The listing builds one solid part. Answer for the finished solid, in the listing's coordinates (mm). A direction names the side the tool comes from. Give positions to 0.01 mm unless a question says otherwise; leave off trailing zeros. Order: outer loops, then holes, each group sorted by start corner. A loop starts at its lowest first (then second) coordinate and runs counter-clockwise, first axis right, second up. Notation, with made-up numbers: (46.25, -27.5) - (50.25, -27.5) arc R22 ccw to (50.25, 8.5) - close; hole circle Ø9 at (13, 47.25). An arc over 180 degrees is marked (long way). Answer as a JSON object with one key per item and string values. Group by question number.
Q1. A cutting plane is placed at B-B, the plane y = 10. Give the vertices of the cut face in (x, z).
Q2. A cutting plane is placed at D-D, the plane y = -5. Give the vertices of the cut face in (x, z).
Q3. The mould has two halves that part along Y. Classify faces 1 (the face through (0, 19, 9)), 2 (the face through (-19.02, -11.06, 3.08)), 3 (the face through (7.706, -4.7, -1.521)): released by +Y, released by -Y, zero draft, split by the parting line, or undercut.
Q4. Given pin 1 (10.5 mm diameter, centred on x = 0, y = 0, fed in from +Z); pin 2 (2 mm diameter, centred on x = 10.5, z = 6.5, fed in from -Y); pin 3 (3.5 mm diameter, centred on y = 17.5, z = 2, fed in from -X); pin 4 (4 mm diameter, centred on y = -8.5, z = 0, fed in from -X), each flat-ended and moving along its own axis, determine where each tip first touches the part or whether it passes through.
Q5. A cutting plane is placed at A-A, the plane z = 7.75. Give the vertices of the cut face in (x, y).
Q6. For faces 4 (the face through (-15, -8, 4)), 5 (the face through (0, 17, 4)), 6 (the face through (-12.906, -13.225, 1.583)), 7 (the face through (-5, 18, 2)), determine the directions among +Z, -Z, +X, -X, +Y, -Y from which every point of the face is accessible in a straight line to the end or side of a thin tool.
Q7. A cutting plane is placed at C-C, the plane x = 0. Give the vertices of the cut face in (y, z), and give its area (3 significant figures).
Q8. Consider line 1 (Y direction, x = 0, z = -0.75); line 2 (Z direction, x = 15.5, y = -5); line 3 (X direction, y = -10.5, z = 3). Determine where each line is inside the solid, lowest interval first.
from build123d import *

# Parameters (mm, degrees)
SKETCH_1_R          = 22
SKETCH_1_R_2        = 17
EXTRUDE_1_DEPTH     = 9
SKETCH_2_R          = 22
EXTRUDE_2_DEPTH     = 3
SKETCH_3_R          = 1
CUT_EXTRUDE_1_DEPTH = 3
CUT_EXTRUDE_2_DEPTH = 25
SKETCH_5_R          = 4
CUT_EXTRUDE_3_DEPTH = 10
FILLET_1_R          = 10
FILLET_2_R          = 10


with BuildPart() as part:
    # 草图1 → 凸台-拉伸1 (new body)
    with BuildSketch(Plane.XY):
        Circle(SKETCH_1_R)
        Circle(SKETCH_1_R_2, mode=Mode.SUBTRACT)
    extrude(amount=EXTRUDE_1_DEPTH)

    # 草图2 → 凸台-拉伸2 (add)
    with BuildSketch(Plane(origin=(0, 0, 0), x_dir=(-1, 0, 0), z_dir=(0, 0, -1))):
        Circle(SKETCH_2_R)
    extrude(amount=EXTRUDE_2_DEPTH)

    # 草图3 → 切除-拉伸1 (cut)
    with BuildSketch(Plane(origin=(0, 0, -3), x_dir=(-1, 0, 0), z_dir=(0, 0, -1))):
        with Locations((0, 10)):
            Circle(SKETCH_3_R)
        with Locations((8.660254038, -5)):
            Circle(SKETCH_3_R)
        with Locations((-8.660254038, -5)):
            Circle(SKETCH_3_R)
    extrude(amount=-CUT_EXTRUDE_1_DEPTH, mode=Mode.SUBTRACT)

    # 草图4 → 切除-拉伸2 (cut)
    with BuildSketch(Plane(origin=(0, 0, -3), x_dir=(-1, 0, 0), z_dir=(0, 0, -1))):
        Polygon((24.787699458, -8.537682263), (5, 2.886751346), (5, 15), (5, 31.006622637), (28.596284234, 19.54376122), align=None)
        Polygon((-6.160254038, -9.330127019), (0, -5.773502692), (19.787699458, -17.197936301), (-4.03507969, -32.43608202), (-23.902747272, -19.573760264), align=None)
        Polygon((-5, 10), (-5, 2.886751346), (-28.902747272, -10.913506226), (-27.638085306, 27.170625695), (-5, 31.006622637), align=None)
    extrude(amount=-CUT_EXTRUDE_2_DEPTH, mode=Mode.SUBTRACT)

    # 草图5 → 切除-拉伸3 (cut)
    with BuildSketch(Plane(origin=(0, 0, -3), x_dir=(-1, 0, 0), z_dir=(0, 0, -1))):
        Circle(SKETCH_5_R)
    extrude(amount=-CUT_EXTRUDE_3_DEPTH, mode=Mode.SUBTRACT)

    # 圆角1
    fillet_1_edges = [part.edges().sort_by_distance(p)[0] for p in [
        (-5, 2.886751346, -1.5),
    ]]
    fillet(fillet_1_edges, radius=FILLET_1_R)

    # 圆角2
    fillet_2_edges = [part.edges().sort_by_distance(p)[0] for p in [
        (5, 2.886751346, -1.5),
        (0, -5.773502692, -1.5),
    ]]
    fillet(fillet_2_edges, radius=FILLET_2_R)


solid = part.part
Reply:
{
 "1": {"outline": "(-5, -3) - (-1, -3) - (-1, 0) - (-5, 0) - close; (1, -3) - (5, -3) - (5, 0) - (1, 0) - close"},
 "2": {"outline": "(-18.66, -3) - (-9.66, -3) - (-9.66, 0) - (-16.25, 0) - (-16.25, 9) - (-18.66, 9) - close; (-7.66, -3) - (7.66, -3) - (7.66, 0) - (-7.66, 0) - close; (9.66, -3) - (18.66, -3) - (18.66, 9) - (16.25, 9) - (16.25, 0) - (9.66, 0) - close"},
 "3": {"face 1": "zero draft", "face 2": "released by -Y", "face 3": "undercut"},
 "4": {"pin 1": "stops at z = 0", "pin 2": "passes through", "pin 3": "stops at x = -5", "pin 4": "stops at x = -21.02"},
 "5": {"outline": "(-21.05, -6.38) arc R22 ccw to (-16.05, -15.04) - (-11.57, -12.45) arc R17 cw to (-16.57, -3.79) - close; (-5, 16.25) arc R17 cw to (5, 16.25) - (5, 21.42) arc R22 ccw to (-5, 21.42) - close; (11.57, -12.45) - (16.05, -15.04) arc R22 ccw to (21.05, -6.38) - (16.57, -3.79) arc R17 cw to start"},
 "6": {"face 4": "+Z, +Y", "face 5": "+Z, -Y", "face 6": "+Z, -Z, -Y", "face 7": "+Z, -Z, -X, +Y"},
 "7": {"outline": "(-7.32, -3) - (-4, -3) - (-4, 0) - (-7.32, 0) - close; (4, -3) - (9, -3) - (9, 0) - (4, 0) - close; (11, -3) - (22, -3) - (22, 9) - (17, 9) - (17, 0) - (11, 0) - close", "area": "103 mm^2"},
 "8": {"line 1": "y = -7.32 to -4, 4 to 9, 11 to 22", "line 2": "z = -3 to 0", "line 3": "x = -19.33 to -13.37, 13.37 to 19.33"}
}
